Check sheet for the modelled part. Datum: model origin and axes. Units: mm. A direction names the side the tool comes from. Give positions to 0.01 mm unless a question says otherwise; leave off trailing zeros. Loops run counter-clockwise (first coordinate to the right, second up) from the corner with the lowest first, then second, coordinate; pieces in that order, holes last. Notation, with made-up numbers: M 17,-0.5 L 29,-0.5 A19 ccw 29,18.5 Z; hole C -24.75,33.25 d3. An arc over 180 degrees is marked long. Write each question's results on one line, items separated by ' | '. Start each with the question number.
1. Sectioned sample at C-C on z = 280. Record the cut outline in (x, y) (3 decimals).
2. Go/stop test with flat-tipped pins: pin 1 (3 mm diameter, centred on x = 12.5, z = 370.5, fed in from +Y) (3 decimals); pin 2 (9.5 mm diameter, centred on x = 0, z = 33.34, fed in from +Y). Record where each tip stops, or that it passes through.
3. Material ranges on line 1 along X through (y, z) = (-2.25, 373) (3 decimals); line 2 along Y through (x, z) = (12, 541.5) (3 decimals); line 3 along X through (y, z) = (-6.5, 607) (3 decimals), recorded low to high.
4. Sectioned sample at A-A on y = 7.5. Record the cut outline in (x, z) (3 decimals), and give its area (3 significant figures).
5. Sectioned sample at B-B on x = 0. Record the cut outline in (y, z) (3 decimals).
6. Tool access check on faces 1 (the flat face through (22.225, 2, 324)), 2 (the flat face through (-25.4, 0, 296)). Record the directions out of +Z, -Z, +X, -X, +Y, -Y that give a thin tool (end or side, any length) a straight path to the whole face; none if there is none.
```python
from build123d import *

# Parameters (mm, degrees)
BOSS_EXTRUDE1_DEPTH = 660.4
CUT_EXTRUDE1_DEPTH  = 662.376201568
CUT_EXTRUDE2_REACH  = 663.376
SKETCH3_R           = 7.9375


with BuildPart() as part:
    # Sketch1 → Boss-Extrude1 (new body)
    with BuildSketch(Plane.XY):
        Polygon((-22.225, -9.525), (-22.225, 12.7), (-25.4, 12.7), (-25.4, -12.7), (25.4, -12.7), (25.4, 12.7), (22.225, 12.7), (22.225, -9.525), align=None)
    extrude(amount=BOSS_EXTRUDE1_DEPTH)

    # Sketch2 → Cut-Extrude1 (cut, through all)
    with BuildSketch(Plane.XZ.offset(12.7)):
        Polygon((25.4, 660.4), (-25.4, 599.858917496), (-25.4, 660.4), align=None)
    extrude(amount=-CUT_EXTRUDE1_DEPTH, mode=Mode.SUBTRACT)

    # Sketch3 → Cut-Extrude2 (cut, up to next)
    with BuildSketch(Plane.XZ.offset(12.7), mode=Mode.PRIVATE) as cut_extrude2_sk1:
        with Locations((0, 33.3375)):
            Circle(SKETCH3_R)
    cut_extrude2_tool1 = extrude(cut_extrude2_sk1.sketch, amount=-CUT_EXTRUDE2_REACH, mode=Mode.PRIVATE) & part.part
    add(cut_extrude2_tool1.solids().sort_by_distance((0, -12.7, 33.3375))[0], mode=Mode.SUBTRACT)


solid = part.part
```
Output values:
1) outline: M -25.4,-12.7 L 25.4,-12.7 L 25.4,12.7 L 22.225,12.7 L 22.225,-9.525 L -22.225,-9.525 L -22.225,12.7 L -25.4,12.7 Z
2) pin 1: y = -9.525 | pin 2: through
3) line 1: -25.4 to -22.225, 22.225 to 25.4 | line 2: -12.7 to -9.525 | line 3: 22.225 to 25.4
4) outline: M -25.4,0 L -22.225,0 L -22.225,603.643 L -25.4,599.859 Z; M 22.225,0 L 25.4,0 L 25.4,660.4 L 22.225,656.616 Z | area: 4,000 mm2
5) outline: M -12.7,0 L -9.525,0 L -9.525,25.4 L -12.7,25.4 Z; M -12.7,41.275 L -9.525,41.275 L -9.525,630.129 L -12.7,630.129 Z
6) face 1: +Z, -Z, +Y | face 2: +Z, -Z, -X, +Y, -Y
